Can you work these out from the model? Positions are in its coordinate system, mm. Face numbers are marked on the shaded views. Give positions to 0.01 mm unless a question says otherwise; leave off trailing zeros. Write each loop counter-clockwise with the first axis right and the second up, starting at its lowest first coordinate (ties: lowest second). Pieces come first, ordered by that corner, then holes. Notation, with made-up numbers: (85, 49.25) - (118, 49.25) arc R20 ccw to (118, 80.25) - close; hole circle Ø8 at (27, -0.75). An arc over 180 degrees is marked (long way). Use a Markdown table: item, result. Add a question column.
```python
from build123d import *

# Parameters (mm, degrees)
BOSS_EXTRUDE1_DEPTH = 1
CUT_EXTRUDE1_REACH  = 31.686
SKETCH5_R           = 0.98
SKETCH2_R           = 3.175
BOSS_EXTRUDE2_DEPTH = 8
BOSS_EXTRUDE3_START = 1.65
SKETCH3_R           = 7.91
BOSS_EXTRUDE3_DEPTH = 1.91
BOSS_EXTRUDE4_REACH = 34.501
SKETCH4_R           = 5


with BuildPart() as part:
    # Sketch1 → Boss-Extrude1 (new body)
    with BuildSketch(Plane.XY):
        Polygon((21.05, -8.2), (21.05, 0), (0, 0), (0, -16.27), (20, -16.27), (24.81, -13), (24.81, -8.2), align=None)
        Polygon((0, -16.27), (0, 0), (-21.05, 0), (-21.05, -8.2), (-24.81, -8.2), (-24.81, -13), (-20, -16.27), align=None)
    extrude(amount=BOSS_EXTRUDE1_DEPTH)

    # Sketch5 → Cut-Extrude1 (cut, up to next)
    with BuildSketch(Plane.XY.offset(1), mode=Mode.PRIVATE) as cut_extrude1_sk1:
        with Locations((-21.7, -9.9)):
            Circle(SKETCH5_R)
    cut_extrude1_tool1 = extrude(cut_extrude1_sk1.sketch, amount=-CUT_EXTRUDE1_REACH, mode=Mode.PRIVATE) & part.part
    # Sketch5 → Cut-Extrude1 (cut, up to next)
    with BuildSketch(Plane.XY.offset(1), mode=Mode.PRIVATE) as cut_extrude1_sk2:
        with Locations((21.7, -9.9)):
            Circle(SKETCH5_R)
    cut_extrude1_tool2 = extrude(cut_extrude1_sk2.sketch, amount=-CUT_EXTRUDE1_REACH, mode=Mode.PRIVATE) & part.part
    add(cut_extrude1_tool1.solids().sort_by_distance((-21.7, -9.9, 1))[0], mode=Mode.SUBTRACT)
    add(cut_extrude1_tool2.solids().sort_by_distance((21.7, -9.9, 1))[0], mode=Mode.SUBTRACT)

    # Sketch2 → Boss-Extrude2 (add)
    with BuildSketch(Plane.XY.offset(1)):
        with Locations((9.55, -4)):
            Circle(SKETCH2_R)
    extrude(amount=BOSS_EXTRUDE2_DEPTH)


with BuildPart() as body_2:
    # Sketch3 → Boss-Extrude3 (new body)
    with BuildSketch(Plane.XY.offset(1).offset(BOSS_EXTRUDE3_START)):
        with Locations(Location((-10.05, -11.5, 0), (0, 0, 180))):
            Circle(SKETCH3_R)
    extrude(amount=BOSS_EXTRUDE3_DEPTH)

    # Sketch4 → Boss-Extrude4 (add, up to next)
    with BuildSketch(Plane.XY.offset(1), mode=Mode.PRIVATE) as boss_extrude4_sk1:
        with Locations(Location((-10.05, -11.5, 0), (0, 0, 252.554012294))):
            Circle(SKETCH4_R)
    boss_extrude4_tool1 = extrude(boss_extrude4_sk1.sketch, amount=BOSS_EXTRUDE4_REACH, mode=Mode.PRIVATE) - body_2.part

    add(part.part)  # Boss-Extrude4 merges part
    add(boss_extrude4_tool1.solids().sort_by_distance((-10.05, -11.5, 1))[0])


solid = body_2.part
```
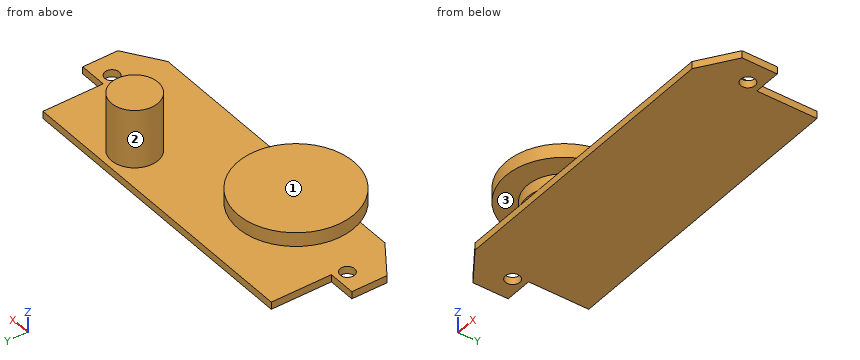
Q1. Suppose I cut it at B-B (x = -10.05). Please give me the cut outline in (y, z), and give its area (3 significant figures).
Q2. Suppose I cut it at C-C (y = -9.9). Please give me the cut outline in (x, z).
Q3. I'm going to push flat-ended pins straight in: P1, Ø1.1, axis at y = -3.5, z = 0.5, coming from the -X side; P2, Ø1, axis at x = 4, z = 2.5, coming from the -Y side; P3, Ø2, axis at x = 9, z = 7.5, coming from the +Y side (3 decimals); P4, Ø8, axis at x = -10.5, y = -15, coming from the +Z side. Where does each tip first touch, or does it pass through?
Q4. Suppose I cut it at A-A (x = -4.5). Please give me the cut outline in (y, z).
Q5. Suppose I cut it at D-D (z = 1.75). Please give me the cut outline in (x, y) (3 decimals).
Q6. If we mould it in two halves opening along Z, with no side actions, what happens to the marked faces 1, 2 and 3? For each: released by +Z, released by -Z, zero draft, split by the parting line, or undercut.
Q7. If I drill on probe 1 along Z at (x, y) = (-13, -5); probe 2 along Z at (x, y) = (-15.5, -4.25); probe 3 along X at (y, z) = (-3.75, 0.75), over which ranges is the centre line in solid material (lowest first)? Write a range as [from, to].
Derived:
| question | item | result |
|---|---|---|
| 1 | outline | (-19.41, 2.65) - (-16.5, 2.65) - (-16.5, 1) - (-16.27, 1) - (-16.27, 0) - (0, 0) - (0, 1) - (-6.5, 1) - (-6.5, 2.65) - (-3.59, 2.65) - (-3.59, 4.56) - (-19.41, 4.56) - close |
| 1 | area | 63.0 mm² |
| 2 | outline | (-24.81, 0) - (-22.68, 0) - (-22.68, 1) - (-24.81, 1) - close; (-20.72, 0) - (20.72, 0) - (20.72, 1) - (-5.31, 1) - (-5.31, 2.65) - (-2.3, 2.65) - (-2.3, 4.56) - (-17.8, 4.56) - (-17.8, 2.65) - (-14.79, 2.65) - (-14.79, 1) - (-20.72, 1) - close; (22.68, 0) - (24.81, 0) - (24.81, 1) - (22.68, 1) - close |
| 3 | P1 | x = -21.05 |
| 3 | P2 | through |
| 3 | P3 | y = -0.825 |
| 3 | P4 | z = 4.56 |
| 4 | outline | (-17.14, 2.65) - (-5.86, 2.65) - (-5.86, 4.56) - (-17.14, 4.56) - close; (-16.27, 0) - (0, 0) - (0, 1) - (-16.27, 1) - close |
| 5 | outline | circle Ø10 at (-10.05, -11.5); circle Ø6.35 at (9.55, -4) |
| 6 | face 1 | released by +Z |
| 6 | face 2 | zero draft |
| 6 | face 3 | undercut |
| 7 | probe 1 | [0, 1], [2.65, 4.56] |
| 7 | probe 2 | [0, 1] |
| 7 | probe 3 | [-21.05, 21.05] |
